The listing builds one solid part. Answer for the finished solid, in the listing's coordinates (mm). A direction names the side the tool comes from. Coordinates: 2 decimals unless noted, no trailing zeros. Loops run counter-clockwise (first coordinate to the right, second up) from the corner with the lowest first, then second, coordinate; pieces in that order, holes last. Notation, with made-up numbers: (-33.75, 30.5) -> (24.25, 30.5) arc R32 cw to (24.25, 59.5) -> close; hole circle Ø3 at (30, 64.25). An arc over 180 degrees is marked (long way). Answer in a Markdown table with one row per item.
Autodesk Fusion 360 part; units mm, degrees
sketch "Sketch1" plane through (0, 0, 0) normal (1, 0, 0) x (0, 1, 0)
  line L0 (-75, 50) -> (13, 50)
  line L1 (13, 50) -> (13, -9)
  line L2 (13, -9) -> (-75, -9)
  line L3 (-75, -9) -> (-75, 50)
  circle A0 centre (-75, 50) radius 2
  circle A1 centre (13, 50) radius 2
  circle A2 centre (-75, -9) radius 2
  circle A3 centre (13, -9) radius 2
  line L4 (-77.5, 52.5) -> (-77.5, 47.5)
  line L5 (-77.5, 47.5) -> (-74, 47.5)
  line L6 (-72.5, 49) -> (-72.5, 52.5)
  line L7 (-72.5, 52.5) -> (10, 52.5)
  line L8 (10, 52.5) -> (10, 49)
  line L9 (11.5, 47.5) -> (15.5, 47.5)
  line L10 (15.5, 47.5) -> (15.5, 52.5)
  line L11 (15.5, 52.5) -> (10, 52.5)
  line L12 (-75, 20.5) -> (-35, 20.5)
  line L13 (-77.5, -11.5) -> (-77.5, -6.5)
  line L14 (-77.5, -6.5) -> (-74, -6.5)
  line L15 (-72.5, -8) -> (-72.5, -11.5)
  line L16 (-72.5, -11.5) -> (10, -11.5)
  line L17 (10, -11.5) -> (10, -8)
  line L18 (11.5, -6.5) -> (15.5, -6.5)
  line L19 (15.5, -6.5) -> (15.5, -11.5)
  line L20 (15.5, -11.5) -> (10, -11.5)
  line L21 (-77.5, 52.5) -> (-72.5, 52.5)
  line L22 (-77.5, 47.5) -> (-77.5, -11.5)
  line L23 (-77.5, -11.5) -> (-72.5, -11.5)
  arc A4 (-74, 47.5) -> (-72.5, 49) centre (-74, 49) ccw
  arc A5 (-72.5, -8) -> (-74, -6.5) centre (-74, -8) ccw
  arc A6 (11.5, -6.5) -> (10, -8) centre (11.5, -8) ccw
  arc A7 (10, 49) -> (11.5, 47.5) centre (11.5, 49) ccw
  line L24 (15.5, 47.5) -> (15.5, -6.5)
  dimension "d1" = 88
  dimension "d2" = 59
  dimension "d3" = 4
  dimension "d4" = 4
  dimension "d5" = 4
  dimension "d6" = 4
  dimension "d7" = 1.5
extrude "Extrude1" add sketch "Sketch1" along normal blind 2 contours L0 L3 A0 L4 L5 L6 L21 | L0 L3 A0 L5 L6 A4 | L0 L6 L7 L8 | L3 L5 L14 L22 | L0 L1 A1 L8 L9 L10 L11 | L0 L1 A1 L8 L9 A7 | L2 L3 A2 L14 L15 A5 | L2 L3 A2 L13 L14 L15 L22 L23 | L1 L9 L18 L24 | L2 L15 L16 L17 | L1 L2 A3 L17 L18 L19 L20 | L1 L2 A3 L17 L18 A6
sketch "Sketch2" plane through (2, 0, 0) normal (1, 0, 0) x (0, 1, 0)
  line L0 (-74, -6.5) -> (-75, -6.5)
  line L1 (-75, -6.5) -> (-75, 47.5)
  line L2 (-75, 47.5) -> (-74, 47.5)
  arc A0 (-74, 47.5) -> (-72.5, 49) centre (-74, 49) ccw
  line L3 (-72.5, 49) -> (-72.5, 50)
  line L4 (-72.5, 50) -> (10, 50)
  line L5 (10, 50) -> (10, 49)
  arc A1 (10, 49) -> (11.5, 47.5) centre (11.5, 49) ccw
  line L6 (11.5, 47.5) -> (13, 47.5)
  line L7 (13, 47.5) -> (13, -6.5)
  line L8 (13, -6.5) -> (11.5, -6.5)
  arc A2 (11.5, -6.5) -> (10, -8) centre (11.5, -8) ccw
  line L9 (10, -8) -> (10, -9)
  line L10 (10, -9) -> (-72.5, -9)
  line L11 (-72.5, -9) -> (-72.5, -8)
  arc A3 (-72.5, -8) -> (-74, -6.5) centre (-74, -8) ccw
  circle A4 centre (13, 50) radius 2
  circle A5 centre (13, -9) radius 2
  circle A6 centre (-75, -9) radius 2
  circle A7 centre (-75, 50) radius 2
  line L12 (15.5, 52.5) -> (-77.5, 52.5)
  line L13 (-77.5, 52.5) -> (-77.5, -11.5)
  line L14 (-77.5, -11.5) -> (15.5, -11.5)
  line L15 (15.5, -11.5) -> (15.5, 52.5)
  line L16 (-75.9596, 48.2453) -> (-77.5, 48.2453)
  line L17 (-73.3661, 51.1535) -> (-73.3661, 52.5)
  line L18 (-76.7298, -7.9961) -> (-77.5, -7.9961)
  line L19 (-73.3661, -10.1535) -> (-73.3661, -11.5)
  line L20 (-60.0421, -9) -> (-60.0421, -11.5)
  line L21 (10, 50) -> (10, 52.5)
  line L22 (0, -11.5) -> (0, -9)
  line L23 (10, -9) -> (10, -11.5)
extrude "Extrude2" add sketch "Sketch2" along normal blind 30 contours L0 L1 L2 A0 L3 L4 L10 L11 A3 A6 A7 L12 L13 L14 L16 L17 L18 L19 L20 L21 | L10 L14 L22 L23
sketch "Sketch3" plane through (0, 0, 50) normal (0, 0, -1) x (1, 0, 0)
  line L0 (0, 72.5) -> (0, -10)
  line L1 (0, -10) -> (2, -10)
  line L2 (2, -10) -> (32, -10)
  line L3 (32, -10) -> (32, 72.5)
  line L4 (32, 72.5) -> (0, 72.5)
  line L5 (32, -10) -> (18, -10)
  line L6 (18, -10) -> (18, -7.5)
  line L7 (18, -7.5) -> (32, -7.5)
  line L8 (32, -7.5) -> (32, -10)
  dimension "d12" = 14
  dimension "d13" = 2.5
extrude "Extrude3" add sketch "Sketch3" along normal up to surface (59 mm away) contours L2 L3 L5 L6 L7 L8
sketch "Sketch4" plane through (0, 0, 0) normal (0, -1, 0) x (1, 0, 0)
  line L0 (2, -9) -> (2, -11.5)
  line L1 (2, -11.5) -> (32, -11.5)
  line L2 (32, -11.5) -> (32, -9)
  line L3 (32, -9) -> (2, -9)
  line L4 (32, -11.5) -> (15, -11.5)
  line L5 (15, -11.5) -> (15, -9)
  line L6 (15, -9) -> (32, -9)
  line L7 (32, -9) -> (32, -11.5)
extrude "Extrude4" add sketch "Sketch4" along normal up to surface (60.0421 mm away) contours L1 L2 L3 L4 L5 L6 L7
sketch "Sketch5" plane through (0, 10, 0) normal (0, 1, 0) x (-1, 0, 0)
  line L0 (-2, -11.5) -> (-2, -9)
  line L1 (-2, -9) -> (-18, -9)
  line L2 (-18, -9) -> (-18, 50)
  line L3 (-18, 50) -> (-2, 50)
  line L4 (-2, 50) -> (-2, 52.5)
  line L5 (-2, 52.5) -> (-32, 52.5)
  line L6 (-32, 52.5) -> (-32, -11.5)
  line L7 (-32, -11.5) -> (-2, -11.5)
  line L8 (-18, 29.9805) -> (-22, 29.9805)
  line L9 (-22, 29.9805) -> (-22, -9)
  line L10 (-22, -9) -> (-18, -9)
extrude "Extrude5" cut sketch "Sketch5" against normal blind 6 contours L2 L8 L9 L10
sketch "Sketch6" plane through (32, 0, 0) normal (1, 0, 0) x (0, 1, 0)
  line L0 (-73.3661, -11.5) -> (10, -11.5)
  line L1 (10, -11.5) -> (10, 52.5)
  line L2 (10, 52.5) -> (-73.3661, 52.5)
  line L3 (-73.3661, 52.5) -> (-73.3661, 51.1535)
  arc A0 (-75.9596, 48.2453) -> (-73.3661, 51.1535) centre (-75, 50) ccw
  line L4 (-75.9596, 48.2453) -> (-77.5, 48.2453)
  line L5 (-77.5, 48.2453) -> (-77.5, -7.9961)
  line L6 (-77.5, -7.9961) -> (-76.7298, -7.9961)
  arc A1 (-73.3661, -10.1535) -> (-76.7298, -7.9961) centre (-75, -9) ccw
  line L7 (-73.3661, -10.1535) -> (-73.3661, -11.5)
  line L8 (7.5, -9) -> (-72.5, -9)
  line L9 (-72.5, -9) -> (-72.5, -8)
  arc A2 (-72.5, -8) -> (-74, -6.5) centre (-74, -8) ccw
  line L10 (-74, -6.5) -> (-75, -6.5)
  line L11 (-75, -6.5) -> (-75, 47.5)
  line L12 (-75, 47.5) -> (-74, 47.5)
  arc A3 (-74, 47.5) -> (-72.5, 49) centre (-74, 49) ccw
  line L13 (-72.5, 49) -> (-72.5, 50)
  line L14 (-72.5, 50) -> (7.5, 50)
  line L15 (7.5, 50) -> (7.5, -9)
  line L16 (-75, 47.5) -> (-73.5326, 47.9393)
  line L17 (-73.5326, 47.9393) -> (-72.7, 50.4)
  line L18 (-72.7, 50.4) -> (9, 51)
  line L19 (9, 51) -> (9, -10.6409)
  line L20 (9, -10.6409) -> (-72.5, -10.6409)
  line L21 (-72.5, -10.6409) -> (-73, -7.5)
  line L22 (-73, -7.5) -> (-74.2896, -6.8066)
  line L23 (-74.2896, -6.8066) -> (-75.5, -6.5)
  line L24 (-75.5, -6.5) -> (-75, 47.5)
extrude "Extrude6" add sketch "Sketch6" against normal blind 2 contours L8 L9 A2 L10 L11 L12 A3 L13 L14 L15
sketch "Sketch7" plane through (32, 0, 0) normal (1, 0, 0) x (0, 1, 0)
  line L0 (-73.3661, -11.5) -> (10, -11.5)
  line L1 (10, -11.5) -> (10, 52.5)
  line L2 (10, 52.5) -> (-73.3661, 52.5)
  line L3 (-73.3661, 52.5) -> (-73.3661, 51.1535)
  arc A0 (-75.9596, 48.2453) -> (-73.3661, 51.1535) centre (-75, 50) ccw
  line L4 (-75.9596, 48.2453) -> (-77.5, 48.2453)
  line L5 (-77.5, 48.2453) -> (-77.5, -7.9961)
  line L6 (-77.5, -7.9961) -> (-76.7298, -7.9961)
  arc A1 (-73.3661, -10.1535) -> (-76.7298, -7.9961) centre (-75, -9) ccw
  line L7 (-73.3661, -10.1535) -> (-73.3661, -11.5)
  circle A2 centre (-31.6831, 20.1246) radius 22.5
  circle A3 centre (-31.6831, 20.1246) radius 18.5
  circle A4 centre (-31.6831, 20.1246) radius 13.5
  circle A5 centre (-31.6831, 20.1246) radius 10.5
  circle A6 centre (-31.6831, 20.1246) radius 5.7443
  line L8 (-34.7796, 42.4105) -> (-31.6831, 20.1246)
  line L9 (-31.6831, 20.1246) -> (-28.1645, 42.3477)
  line L10 (-31.6831, 20.1246) -> (-35.2016, -2.0986)
  line L11 (-31.6831, 20.1246) -> (-27.4785, -1.9791)
  dimension "d22" = 45
  dimension "d23" = 37
  dimension "d24" = 27
  dimension "d25" = 21
extrude "Extrude7" cut sketch "Sketch7" against normal blind 4 contours A2 A3 L9 L11 | A2 A3 L8 L10 | A4 A5 L9 L11 | A4 A5 L8 L10
extrude "Extrude8" cut 1 faces at (19.3333, 9.1667, 29.9805) along direction (0, 0, 1) blind 20
Item 1: A cutting plane is placed at A-A, the plane z = 46.5. Determine the outline of the cut face in (x, y), plus the area to 3 significant figures.
Findings below:
| item | result |
|---|---|
| outline | (0, -77.5) -> (32, -77.5) -> (32, 10) -> (22, 10) -> (22, 7.5) -> (30, 7.5) -> (30, -75) -> (0, -75) -> close; (0, 13) -> (2, 13) -> (2, 15.5) -> (0, 15.5) -> close |
| area | 275 mm2 |
Item 2: Find the intervals of material crossed by probe 1 along Z at (x, y) = (27.5, -8); probe 2 along Y at (x, z) = (29, 42); probe 3 along Y at (x, z) = (12.5, -4.5), in increasing order.
Findings below:
| item | result |
|---|---|
| probe 1 | z = -11.5 to -9, 50 to 52.5 |
| probe 2 | y = -77.5 to -75, 7.5 to 10 |
| probe 3 | y = -77.5 to -75 |
Item 3: A tool of negligible diameter and unlimited length cuts with its end or side. For faces 4 (the face through (15, -75, 20)), 5 (the face through (20, 9, 49.98)), 6 (the face through (31.014, -21.183, 20.082)), from which of +Z, -Z, +X, -X, +Y, -Y can it reach the whole face along a straight path? Write none if from no direction.
Findings below:
| item | result |
|---|---|
| face 4 | -X |
| face 5 | -X, +Y |
| face 6 | +X, -X |
Item 4: A cutting plane is placed at B-B, the plane y = -6.5. Determine the outline of the cut face in (x, z).
Findings below:
| item | result |
|---|---|
| outline | (0, -11.5) -> (2, -11.5) -> (2, -9) -> (0, -9) -> close; (0, 50) -> (30, 50) -> (30, -9) -> (15, -9) -> (15, -11.5) -> (32, -11.5) -> (32, 52.5) -> (0, 52.5) -> close |
Item 5: A cutting plane is placed at C-C, the plane y = 3.5. Determine the outline of the cut face in (x, z).
Findings below:
| item | result |
|---|---|
| outline | (0, -11.5) -> (32, -11.5) -> (32, 52.5) -> (0, 52.5) -> (0, 50) -> (30, 50) -> (30, -9) -> (0, -9) -> close |
Item 6: Determine the mould class of faces 1 (the face through (22, 9, 21)), 2 (the face through (15, -30, -10)), 3 (the face through (1, 15.5, 20)) for opening direction Y: +Y half, -Y half, draft (parallel to the pull), parting line (faces both ways), or undercut.
Findings below:
| item | result |
|---|---|
| face 1 | draft |
| face 2 | undercut |
| face 3 | +Y half |
Item 7: Flat-ended cylindrical pins translate along their axes: pin 1 Ø0.5 at (x, z) = (22, -8.5) entering from +Y; pin 2 Ø1.5 at (x, z) = (20, -11) entering from -Y; pin 3 Ø1.6 at (y, z) = (13.5, 24.5) entering from +X. Find the tip coordinate at first contact, or state that the pin passes through.
Findings below:
| item | result |
|---|---|
| pin 1 | stops at y = 10 |
| pin 2 | stops at y = -73.37 |
| pin 3 | stops at x = 2 |
